Source: CAD feature listing. Evaluate the final solid. Frame: model axes, mm. Face numbers are marked on the shaded views. A direction names the side the tool comes from. Round coordinates to 2 decimals unless told otherwise and drop trailing zeros. Order: outer loops, then holes, each group sorted by start corner. A loop starts at its lowest first (then second) coordinate and runs counter-clockwise, first axis right, second up. Notation, with made-up numbers: (89, 32) -> (98, 32) arc R31 ccw to (98, 66) -> close; hole circle Ø2 at (52, -21). An arc over 180 degrees is marked (long way). Answer as CSV lines item,"result".
from build123d import *

# Parameters (mm, degrees)
CYLINDER026_R     = 1.25
CYLINDER026_DEPTH = 10
CYLINDER027_W     = 4
CYLINDER027_H     = 26
CYLINDER027_ANGLE = 180
BOX029_W          = 28
BOX029_H          = 2.75
BOX029_DEPTH      = 2


with BuildPart() as b_no001:
    # Cylinder026 → Cylinder026 (new body)
    with BuildSketch(Plane(origin=(55, 29, 4), x_dir=(1, 0, 0), z_dir=(0, 0, 1))):
        Circle(CYLINDER026_R)
    extrude(amount=CYLINDER026_DEPTH)


with BuildPart() as s015:
    # Cylinder027 → Cylinder027 (revolve)
    with BuildSketch(Plane(origin=(55, 28, -14), x_dir=(1, 0, 0), z_dir=(0, -1, 0))):
        with Locations((2, 13)):
            Rectangle(CYLINDER027_W, CYLINDER027_H)
    revolve(axis=Axis((55, 28, -14), (0, 0, 1)), revolution_arc=CYLINDER027_ANGLE)


with BuildPart() as obj1:
    # Box029 → Box029 (new body)
    with BuildSketch(Plane(origin=(33, 25.25, 10), x_dir=(1, 0, 0), z_dir=(0, 0, 1))):
        with Locations((14, 1.375)):
            Rectangle(BOX029_W, BOX029_H)
    extrude(amount=BOX029_DEPTH)

    # Fusion: union S015
    add(s015.part)

    # Cut010: cut B_NO001
    add(b_no001.part, mode=Mode.SUBTRACT)


with BuildPart() as obj1_1:
    # Cut010 placement: moved
    add(obj1.part.moved(Location((9, 15, 0))))


solid = obj1_1.part
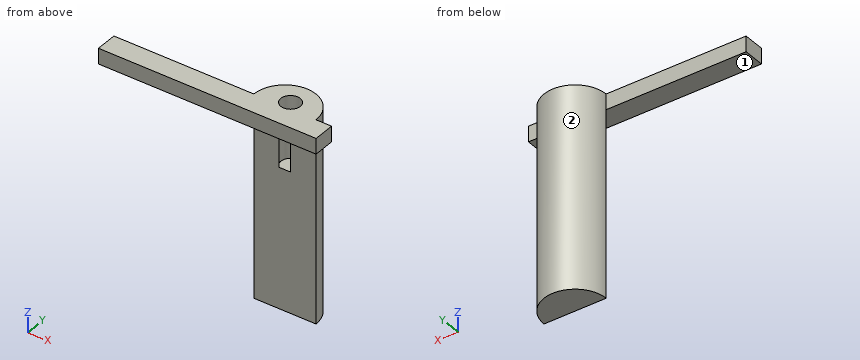
1. Section query B-B on y = 44.75. Return loops of the section in (x, z).
Results below:
outline,"(60.4, -14) -> (67.6, -14) -> (67.6, 12) -> (65, 12) -> (65, 4) -> (63, 4) -> (63, 12) -> (60.4, 12) -> close"
2. Line query: L1, parallel to X at y = 44, z = 6.5; L2, parallel to Z at x = 56.25, y = 42; L3, parallel to Y at x = 64, z = 9.25. Output: solid intervals per line, ascending. Write a range as [from, to].
Results below:
L1,"[60.13, 62.75], [65.25, 67.87]"
L2,"[10, 12]"
L3,"[45.25, 47]"
3. Reachability of the marked faces 1 and 2 from +Z, -Z, +X, -X, +Y, -Y: full face, straight path, thin tool, end or side. Return the list, or none.
Results below:
face 1,"-Z, +X, -X, -Y"
face 2,"+Z, -Z, +Y"
4. Section query C-C on z = 1.75. Return loops of the section in (x, y), and give its area (3 significant figures).
Results below:
outline,"(60, 43) -> (68, 43) arc R4 ccw to start"
area,"25.1 mm2"
5. Pin query (flat end, axial travel): pin 1 (6.5 mm diameter, centred on x = 65, z = -3, fed in from -Y); pin 2 (0.6 mm diameter, centred on x = 68.5, z = 11, fed in from +Y); pin 3 (1.8 mm diameter, centred on x = 63.5, y = 44, fed in from +Z); pin 4 (3 mm diameter, centred on y = 42, z = -2.5, fed in from +X). Return the tip coordinate at first contact, or that it passes through.
Results below:
pin 1,"y = 43"
pin 2,"y = 43"
pin 3,"z = 12"
pin 4,"x = 68"
6. Section query D-D on x = 44. Return loops of the section in (y, z).
Results below:
outline,"(40.25, 10) -> (43, 10) -> (43, 12) -> (40.25, 12) -> close"
7. Section query A-A on x = 64. Return loops of the section in (y, z), and give its area (3 significant figures).
Results below:
outline,"(40.25, 10) -> (42.75, 10) -> (42.75, 12) -> (40.25, 12) -> close; (43, -14) -> (47, -14) -> (47, 12) -> (45.25, 12) -> (45.25, 4) -> (43, 4) -> close"
area,"91.0 mm2"
